```python
from build123d import *

# Parameters (mm, degrees)
BOSS_EXTRUDE1_DEPTH          = 18
SKETCH2_R                    = 1
CUT_EXTRUDE1_DEPTH           = 18
F_5_0_5_DIAMETER_HOLE1_D     = 5
F_5_0_5_DIAMETER_HOLE2_D     = 5
F_8_0_8_DIAMETER_HOLE1_D     = 8
F_8_0_8_DIAMETER_HOLE1_DEPTH = 26


with BuildPart() as part:
    # Sketch1 → Boss-Extrude1 (new body)
    with BuildSketch(Plane.XY):
        Polygon((200, 234), (124, 234), (124, 303), (79, 303), (79, 365), (124, 365), (124, 434), (0, 434), (0, 0), (200, 0), align=None)
    extrude(amount=BOSS_EXTRUDE1_DEPTH)

    # Sketch2 → Cut-Extrude1 (cut)
    with BuildSketch(Plane.XY.offset(18)):
        with Locations((79, 365)):
            Circle(SKETCH2_R)
        with Locations((79, 303)):
            Circle(SKETCH2_R)
        with Locations((124, 234)):
            Circle(SKETCH2_R)
    extrude(amount=-CUT_EXTRUDE1_DEPTH, mode=Mode.SUBTRACT)

    # Ø5.0 (5) Diameter Hole1 (through all)
    with Locations(Plane.XY.offset(18)):
        with Locations((9, 397), (9, 277), (9, 157), (9, 37)):
            Hole(F_5_0_5_DIAMETER_HOLE1_D / 2)

    # Ø5.0 (5) Diameter Hole2 (through all)
    with Locations(Plane(origin=(0, 0, 0), x_dir=(-1, 0, 0), z_dir=(0, 0, -1))):
        with Locations((-191, 202), (-191, 117), (-191, 32)):
            Hole(F_5_0_5_DIAMETER_HOLE2_D / 2)

    # Ø8.0 (8) Diameter Hole1
    with Locations(Plane(origin=(124, 0, 0), x_dir=(0, 0, -1), z_dir=(1, 0, 0))):
        with Locations((-9, 398), (-9, 270)):
            Hole(F_8_0_8_DIAMETER_HOLE1_D / 2, depth=F_8_0_8_DIAMETER_HOLE1_DEPTH)


solid = part.part
```
Design review of the part built by this model. Coordinates are the model's own, in mm. A direction names the side the tool comes from. Give positions to 0.01 mm unless a question says otherwise; leave off trailing zeros. Order: outer loops, then holes, each group sorted by start corner. A loop starts at its lowest first (then second) coordinate and runs counter-clockwise, first axis right, second up. Notation, with made-up numbers: (-1, 89) - (16, 89) arc R18 ccw to (16, 119) - close; hole circle Ø10 at (78, -16). An arc over 180 degrees is marked (long way). Use a Markdown table: item, result. Add a question column.
(1) Add section A-A on z = 9. Give the boundary of the cut face in (x, y), then the cut area to 3 significant figures.
(2) Mouldability with a two-part tool opening along Z and no side actions: class faces 6 (the face through (76, 172, 18)), 7 (the face through (200, 115, 9)), 8 (the face through (98, 398, 9)), 9 (the face through (76, 172, 0)) as +Z half, -Z half, draft (parallel to the pull), parting line (faces both ways), or undercut.
(3) Clearance check with flat-ended pins moving along their axes: P1, Ø1, axis at x = 126.5, z = 4.5, coming from the +Y side; P2, Ø4, axis at y = 315, z = 16, coming from the +X side; P3, Ø4, axis at x = 9, y = 277, coming from the +Z side; P4, Ø1, axis at y = 296, z = 7.5, coming from the +X side. State where each tip first meets the part, or that it passes through.
(4) Machinability: for faces 1 (the face through (98, 270, 9)), 2 (the face through (99, 0, 9)), 3 (the face through (102, 303, 9)), 4 (the face through (124, 268.5, 12.9)), 5 (the face through (63, 434, 9)), which of the approach directions +Z, -Z, +X, -X, +Y, -Y give a long, thin tool a straight path to every point of the face, cutting with its end or side? Answer none if there is none.
(5) Add section C-C on y = 330.5. Give the boundary of the cut face in (x, z).
(6) Wall thickness on probe 1 along Y at (x, z) = (9, 4); probe 2 along Z at (x, y) = (104.5, 270); probe 3 along X at (y, z) = (202, 5.5): over which ranges is each line inside the solid? List them lowest first. Write a range as [from, to].
(7) Add section D-D on x = 171. Give the boundary of the cut face in (y, z), then the cut area to 3 significant figures.
(8) Add section B-B on x = 92. Give the boundary of the cut face in (y, z), then the cut area to 3 significant figures.
Report:
| question | item | result |
|---|---|---|
| 1 | outline | (0, 0) - (200, 0) - (200, 234) - (125, 234) arc R1 cw (long way) to (124, 235) - (124, 266) - (98, 266) - (98, 274) - (124, 274) - (124, 303) - (80, 303) arc R1 cw (long way) to (79, 304) - (79, 364) arc R1 cw (long way) to (80, 365) - (124, 365) - (124, 394) - (98, 394) - (98, 402) - (124, 402) - (124, 434) - (0, 434) - close; hole circle Ø5 at (9, 37); hole circle Ø5 at (9, 157); hole circle Ø5 at (9, 277); hole circle Ø5 at (9, 397); hole circle Ø5 at (191, 32); hole circle Ø5 at (191, 117); hole circle Ø5 at (191, 202) |
| 1 | area | 68,200 mm² |
| 2 | face 6 | +Z half |
| 2 | face 7 | draft |
| 2 | face 8 | undercut |
| 2 | face 9 | -Z half |
| 3 | P1 | stops at y = 234 |
| 3 | P2 | stops at x = 79 |
| 3 | P3 | passes through |
| 3 | P4 | stops at x = 124 |
| 4 | face 1 | +X |
| 4 | face 2 | +Z, -Z, +X, -X, -Y |
| 4 | face 3 | +Z, -Z, +X |
| 4 | face 4 | +Z, -Z, +X, +Y |
| 4 | face 5 | +Z, -Z, +X, -X, +Y |
| 5 | outline | (0, 0) - (79, 0) - (79, 18) - (0, 18) - close |
| 6 | probe 1 | y = [0, 34.5], [39.5, 154.5], [159.5, 274.5], [279.5, 394.5], [399.5, 434] |
| 6 | probe 2 | z = [0, 5], [13, 18] |
| 6 | probe 3 | x = [0, 188.5], [193.5, 200] |
| 7 | outline | (0, 0) - (234, 0) - (234, 18) - (0, 18) - close |
| 7 | area | 4,210 mm² |
| 8 | outline | (0, 0) - (303, 0) - (303, 18) - (0, 18) - close; (365, 0) - (434, 0) - (434, 18) - (365, 18) - close |
| 8 | area | 6,700 mm² |
